```python
from build123d import *

# Parameters (mm, degrees)
BOSS_EXTRUDE1_DEPTH = 10
CIRPATTERN1_COUNT   = 2
CIRPATTERN1_ANGLE   = 90
SKETCH4_R           = 2
SKETCH4_R_2         = 9
BOSS_EXTRUDE2_DEPTH = 3


with BuildPart() as part:
    # Sketch1 → Boss-Extrude1 (new body)
    with BuildSketch(Plane(origin=(0, 0, 0), x_dir=(1, 0, 0), z_dir=(0, 1, 0))):
        with BuildLine():
            Line((0, 15), (-26.900155428, 6.278700475))
            Line((-26.900155428, 6.278700475), (-37.47437809, 2.750369919))
            Line((-37.47437809, 2.750369919), (-36.958650594, -0.903972442))
            Line((-36.958650594, -0.903972442), (-26.900155428, 3.317423045))
            Line((-26.900155428, 3.317423045), (-2.821131559, 11.193160892))
            ThreePointArc((-2.821131559, 11.193160892), (11.303828334, 2.338610491), (1.8517881, -11.393705054))
            Line((1.8517881, -11.393705054), (-25.145499842, -12.903972442))
            Line((-25.145499842, -12.903972442), (-32.586903668, -12.903972442))
            Line((-32.586903668, -12.903972442), (-36.958650594, -12.903972442))
            Line((-36.958650594, -12.903972442), (-36.958650594, -15.903972442))
            Line((-36.958650594, -15.903972442), (-0.325723138, -14.996463064))
            ThreePointArc((-0.325723138, -14.996463064), (14.99911574, -0.16287117), (0, 15))
        make_face()
    boss_extrude1 = extrude(amount=BOSS_EXTRUDE1_DEPTH)

    # CirPattern1: Boss-Extrude1 ×2 about axis
    cirpattern1_axis = Axis((-31.052075218, 5, 0), (0, 0, -1))
    for i in range(1, CIRPATTERN1_COUNT):
        add(boss_extrude1.rotate(cirpattern1_axis, i * CIRPATTERN1_ANGLE / (CIRPATTERN1_COUNT - 1)))

    # Sketch4 → Boss-Extrude2 (add)
    with BuildSketch(Plane(origin=(0, 0, 12.903972442), x_dir=(-1, 0, 0), z_dir=(0, 0, -1))):
        Polygon((25.145499842, 5), (29.689369088, -0.906575376), (4.282629912, -20.451725217), (20.145121552, -41.071377206), (-6.070129591, -61.238507201), (-36.557141793, -21.608441758), (-10.34189065, -1.441311764), (-0.261239334, -14.545149841), align=None)
        with Locations((-13.91810605, -12.988615209)):
            Circle(SKETCH4_R, mode=Mode.SUBTRACT)
        with Locations((7.422802492, -40.729661018)):
            Circle(SKETCH4_R, mode=Mode.SUBTRACT)
        with Locations((-9.58846225, -31.737060066)):
            Circle(SKETCH4_R_2, mode=Mode.SUBTRACT)
    extrude(amount=-BOSS_EXTRUDE2_DEPTH)


solid = part.part
```
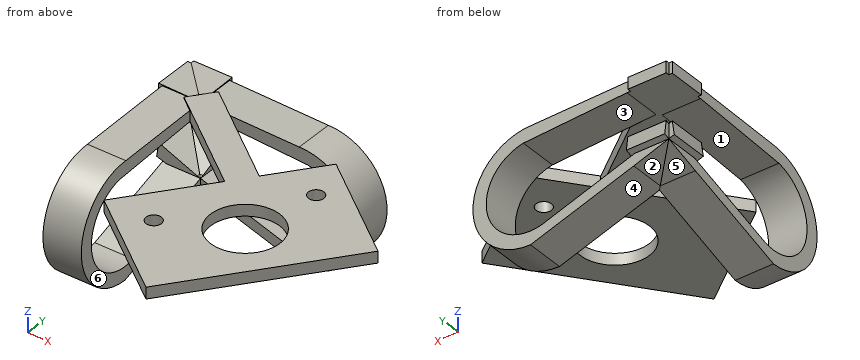
Can you work these out from the model? Positions are in its coordinate system, mm. Face numbers are marked on the shaded views. A direction names the side the tool comes from. Give positions to 0.01 mm unless a question says otherwise; leave off trailing zeros. Loops run counter-clockwise (first coordinate to the right, second up) from the corner with the lowest first, then second, coordinate; pieces in that order, holes last. Notation, with made-up numbers: M -23,56 L 18,56 A25 ccw 18,95 Z; hole C -4,45 d8. An arc over 180 degrees is marked long. One line per question, with ' | ' between items. Start each with the question number.
Q1. If I drill on line 1 (Z direction, x = 6.5, y = -10); line 2 (Z direction, x = -27.5, y = -11); line 3 (Z direction, x = -30.5, y = -21), over which ranges is the centre line in solid material (lowest first)? Write a range as from..to.
Q2. If we mould it in two halves opening along X, with no side actions, what happens to the marked faces 4, 5 and 6? For each: +X half, -X half, draft (parallel to the pull), parting line (faces both ways), or undercut.
Q3. If we section it at A-A (y = -30): Please give me the cut outline in (x, z), plus the area to 3 significant figures.
Q4. For pin 1 Ø4 at (x, y) = (16, -14) entering from -Z; pin 2 Ø12 at (y, z) = (-27, -8) entering from -X; pin 3 Ø3.5 at (x, y) = (13.92, -12.99) entering from +Z; pin 4 Ø5 at (x, z) = (-31.5, -2) entering from -Y, each with a flat end and sliding along its axis, tell me the tip position at first contact or that it passes through.
Q5. For the marked faces 1, 2 and 3, which set-ups out of +Z, -Z, +X, -X, +Y, -Y let a thin tool reach every point of the face, with its end or its side?
Q6. If we section it at B-B (x = 4): Please give me the cut outline in (y, z), plus the area to 3 significant figures.
Q7. If we section it at C-C (z = 7): Please give me the cut outline in (x, y).
Q8. If we section it at D-D (x = 26): Please give me the cut outline in (y, z), plus the area to 3 significant figures.
Computed:
1) line 1: z = 12.9..15.9 | line 2: z = -10.12..-7.19, 12.34..15.36 | line 3: z = -13.36..-10.46, 11.78..15.11
2) face 4: -X half | face 5: draft | face 6: undercut
3) outline: M -36.05,-14.47 L -26.05,-14.47 L -26.05,-10.85 L -36.05,-10.85 Z; M -36.05,10.85 L -26.05,10.85 L -26.05,14.47 L -36.05,14.47 Z; M -11.63,12.9 L 0.76,12.9 L 0.76,15.9 L -11.63,15.9 Z; M 18.42,12.9 L 30.1,12.9 L 30.1,15.9 L 18.42,15.9 Z | area: 145 mm²
4) pin 1: stops at z = 12.9 | pin 2: stops at x = -36.05 | pin 3: passes through | pin 4: stops at y = -41.05
5) face 1: +X, -X, +Y | face 2: -Z, -X, +Y | face 3: -X, +Y, -Y
6) outline: M -59.65,12.9 L -38.79,12.9 L -38.79,15.9 L -59.65,15.9 Z; M -24.68,12.9 L -9.69,12.9 L -9.69,15.9 L -24.68,15.9 Z; M 0,-14.46 L 10,-14.46 L 10,-10.83 L 0,-10.83 Z; M 0,10.83 L 10,10.83 L 10,14.46 L 0,14.46 Z | area: 180 mm²
7) outline: M -36.05,-39.32 L -26.05,-39.32 L -26.05,-35.23 L -36.05,-35.23 Z; M 9.18,0 L 13.27,0 L 13.27,10 L 9.18,10 Z
8) outline: M -35.33,12.9 L -13.49,12.9 L -13.49,15.9 L -35.33,15.9 Z | area: 65.5 mm²
